Check sheet for the modelled part. Datum: model origin and axes. Units: mm. Face numbers are marked on the shaded views. A direction names the side the tool comes from. Give positions to 0.01 mm unless a question says otherwise; leave off trailing zeros. Write each loop counter-clockwise with the first axis right and the second up, starting at its lowest first coordinate (ties: lowest second). Pieces come first, ordered by that corner, then holes. Notation, with made-up numbers: (67.25, 65.5) -> (98.25, 65.5) arc R25 ccw to (98.25, 85.5) -> close; hole circle Ø4 at (40, -10.5). An arc over 180 degrees is marked (long way). Answer as a JSON object with one key per item and string values.
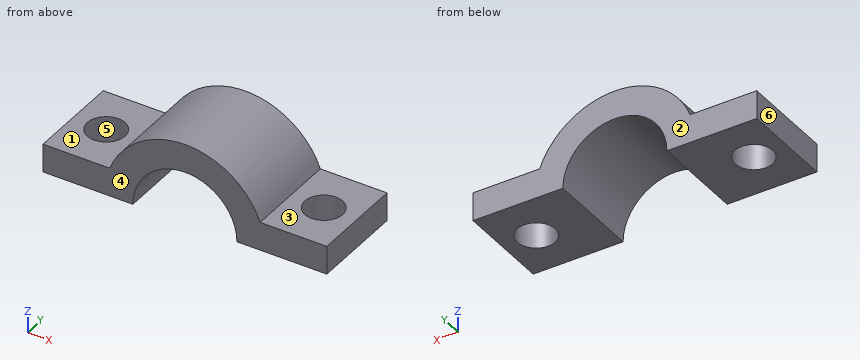
from build123d import *

# Parameters (mm, degrees)
F0_W     = 30
F0_H     = 10
F1_DEPTH = 17
F3_DEPTH = 25
F4_R     = 2
F5_DEPTH = 25


with BuildPart() as f1:
    # F0 (on Top) → F1 (new body)
    with BuildSketch(Plane.XY):
        with Locations((5.848114, 1.410811)):
            Rectangle(F0_W, F0_H)
    extrude(amount=F1_DEPTH)

    # F2 (on face) → F3 (cut)
    with BuildSketch(Plane.XZ.offset(3.589189)):
        with BuildLine():
            ThreePointArc((-2.104872, 3), (5.848114, 8.5), (13.801101, 3))
            Line((13.801101, 3), (20.848114, 3))
            Line((20.848114, 3), (20.848114, 17))
            Line((20.848114, 17), (-9.151886, 17))
            Line((-9.151886, 17), (-9.151886, 3))
            Line((-9.151886, 3), (-2.104872, 3))
        make_face()
        with BuildLine():
            Line((0.348114, 0), (11.348114, 0))
            ThreePointArc((11.348114, 0), (5.848114, 5.5), (0.348114, 0))
        make_face()
    extrude(amount=-F3_DEPTH, mode=Mode.SUBTRACT)

    # F4 (on face) → F5 (cut)
    with BuildSketch(Plane.XY.offset(3)):
        with Locations((-5.651886, 1.410811)):
            Circle(F4_R)
        with Locations((17.348114, 1.410811)):
            Circle(F4_R)
    extrude(amount=-F5_DEPTH, mode=Mode.SUBTRACT)


solid = f1.part
1. Sectioned sample at A-A, the plane z = 2.5. Enter the section's corners in (x, y).
Determined:
{"outline": "(-9.15, -3.59) -> (0.95, -3.59) -> (0.95, 6.41) -> (-9.15, 6.41) -> close; (10.75, -3.59) -> (20.85, -3.59) -> (20.85, 6.41) -> (10.75, 6.41) -> close; hole circle Ø4 at (-5.65, 1.41); hole circle Ø4 at (17.35, 1.41)"}
2. Access from +Z, -Z, +X, -X, +Y, -Y to the whole of each face (thin tool, end or side, straight path). Record for the marked faces 1, 2 and 3.
Determined:
{"face 1": "+Z, -X, +Y, -Y", "face 2": "+Z, -Z, +X, -X, +Y", "face 3": "+Z, +X, +Y, -Y"}
3. Sectioned sample at C-C, the plane x = -7. Enter the section's corners in (y, z).
Determined:
{"outline": "(-3.59, 0) -> (-0.07, 0) -> (-0.07, 3) -> (-3.59, 3) -> close; (2.89, 0) -> (6.41, 0) -> (6.41, 3) -> (2.89, 3) -> close"}
4. Sectioned sample at B-B, the plane y = 2. Enter the section's corners in (x, z).
Determined:
{"outline": "(-9.15, 0) -> (-7.56, 0) -> (-7.56, 3) -> (-9.15, 3) -> close; (-3.74, 0) -> (0.35, 0) arc R5.5 cw to (11.35, 0) -> (15.44, 0) -> (15.44, 3) -> (13.8, 3) arc R8.5 ccw to (-2.1, 3) -> (-3.74, 3) -> close; (19.26, 0) -> (20.85, 0) -> (20.85, 3) -> (19.26, 3) -> close"}
5. Sectioned sample at D-D, the plane y = 4. Enter the section's corners in (x, z).
Determined:
{"outline": "(-9.15, 0) -> (0.35, 0) arc R5.5 cw to (11.35, 0) -> (20.85, 0) -> (20.85, 3) -> (13.8, 3) arc R8.5 ccw to (-2.1, 3) -> (-9.15, 3) -> close"}
6. Mould release check, pull along Y, two halves, no side actions. Record for the marked faces 4, 5 and 6: released by +Y, released by -Y, zero draft, split by the parting line, or undercut.
Determined:
{"face 4": "released by -Y", "face 5": "undercut", "face 6": "zero draft"}
7. Scan lines: L1, parallel to Y at x = -5.75, z = 0.5; L2, parallel to X at y = 3, z = 2.75; L3, parallel to Y at x = -4.5, z = 2.5. Record each from-to range of solid material in increasing order. Write a range as [from, to].
Determined:
{"L1": "[-3.59, -0.59], [3.41, 6.41]", "L2": "[-9.15, -6.87], [-4.44, 1.08], [10.61, 16.13], [18.56, 20.85]", "L3": "[-3.59, -0.22], [3.05, 6.41]"}
8. Go/stop test with flat-tipped pins: P1, Ø5, axis at y = 2, z = 7, coming from the +X side; P2, Ø5.5, axis at x = 17, y = 1, coming from the +Z side; P3, Ø2, axis at y = -1.5, z = 4.5, coming from the -X side; P4, Ø2, axis at x = -6.5, y = 1.5, coming from the +Z side. Record where each tip stops, or that it passes through.
Determined:
{"P1": "x = 13.06", "P2": "z = 3", "P3": "x = -1.9", "P4": "through"}
